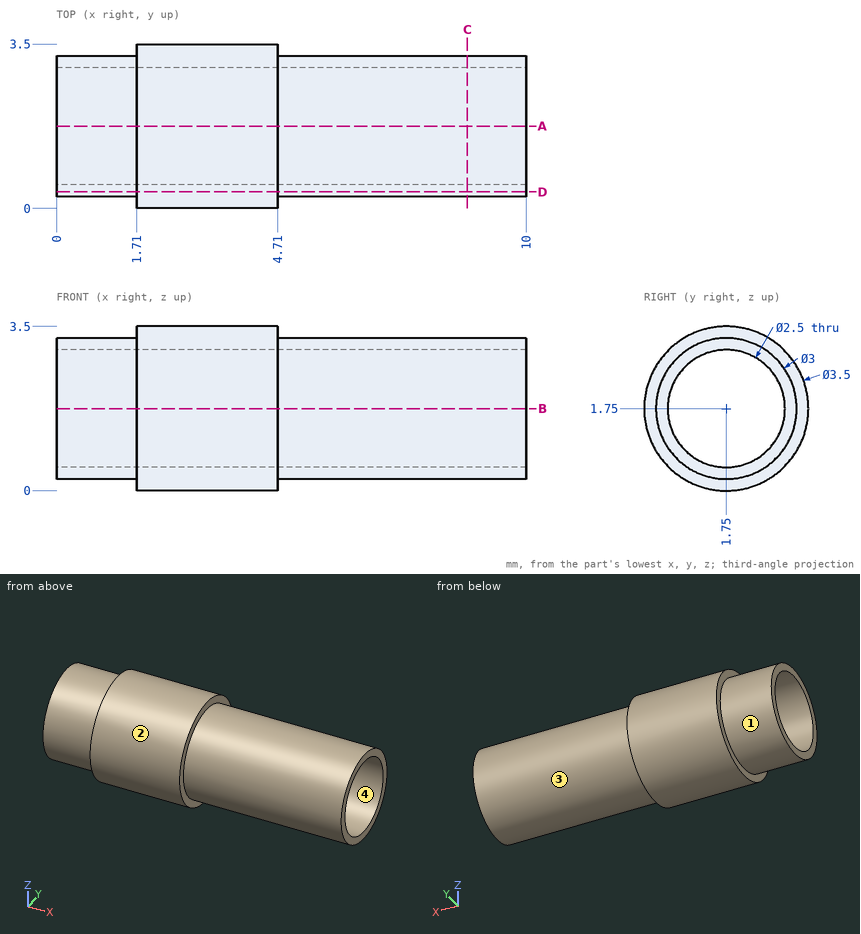
Check sheet for the drawn part. Datum: minimum x, y, z corner. Units: mm. A direction names the side the tool comes from. Give positions to 0.01 mm unless a question says otherwise; leave off trailing zeros. Order: outer loops, then holes, each group sorted by start corner. A loop starts at its lowest first (then second) coordinate and runs counter-clockwise, first axis right, second up. Notation, with made-up numbers: (-24.75, 6.25) - (22.25, 6.25) arc R25 ccw to (22.25, 40.25) - close; hole circle Ø1 at (58.5, 78.25). An arc over 180 degrees is marked (long way). Write item = value, one per line. Start each with the question number.
1) Section check A-A (y = 1.75). Enter the section's corners in (x, z), then the cut area to 3 significant figures.
2) Gauge pin test, flat ends, axial feed: pin 1 Ø2 at (x, z) = (8, 3) entering from -Y; pin 2 Ø2 at (x, y) = (8.5, 1.5) entering from +Z. Record the tip position at first contact, or that the pin passes through.
3) Access from +Z, -Z, +X, -X, +Y, -Y to the whole of each face (thin tool, end or side, straight path). Record for the marked faces 1 and 2.
4) Scan lines: L1, parallel to Z at x = 4, y = 1.75; L2, parallel to Z at x = 5.75, y = 1.75; L3, parallel to X at y = 0.9, z = 0.4. Record each from-to range of solid material in increasing order.
5) Section check D-D (y = 0.35). Enter the section's corners in (x, z), then the cut area to 3 significant figures.
6) Section check C-C (x = 8.75). Enter the section's corners in (y, z).
7) Draft check along Z on the marked faces 3 and 4. Enter one of: released by +Z, released by -Z, zero draft, split by the parting line, or undercut.
Geometry check:
q1.outline = (0, 0.25) - (1.71, 0.25) - (1.71, 0) - (4.71, 0) - (4.71, 0.25) - (10, 0.25) - (10, 0.5) - (0, 0.5) - close; (0, 3) - (10, 3) - (10, 3.25) - (4.71, 3.25) - (4.71, 3.5) - (1.71, 3.5) - (1.71, 3.25) - (0, 3.25) - close
q1.area = 6.50 mm2
q2.pin_1 = 0.27
q2.pin_2 = 3.25
q3.face_1 = -X
q3.face_2 = +X, -X
q4.L1 = 0 to 0.5, 3 to 3.5
q4.L2 = 0.25 to 0.5, 3 to 3.25
q4.L3 = 1.71 to 4.71
q5.outline = (0, 1.21) - (1.71, 1.21) - (1.71, 0.7) - (4.71, 0.7) - (4.71, 1.21) - (10, 1.21) - (10, 2.29) - (4.71, 2.29) - (4.71, 2.8) - (1.71, 2.8) - (1.71, 2.29) - (0, 2.29) - close
q5.area = 13.8 mm2
q6.outline = circle Ø3 at (1.75, 1.75); hole circle Ø2.5 at (1.75, 1.75)
q7.face_3 = split by the parting line
q7.face_4 = undercut
